Work out the finished part from the listing and answer in its coordinate system (mm). Face numbers are marked on the shaded views. A direction names the side the tool comes from. Give positions to 0.01 mm unless a question says otherwise; leave off trailing zeros. Loops run counter-clockwise (first coordinate to the right, second up) from the corner with the lowest first, then second, coordinate; pieces in that order, holes last. Notation, with made-up numbers: M 63,22 L 93,22 A24 cw 93,43 Z; hole C 13.25,31.5 d6. An arc over 180 degrees is marked long. Use a Markdown table: item, result.
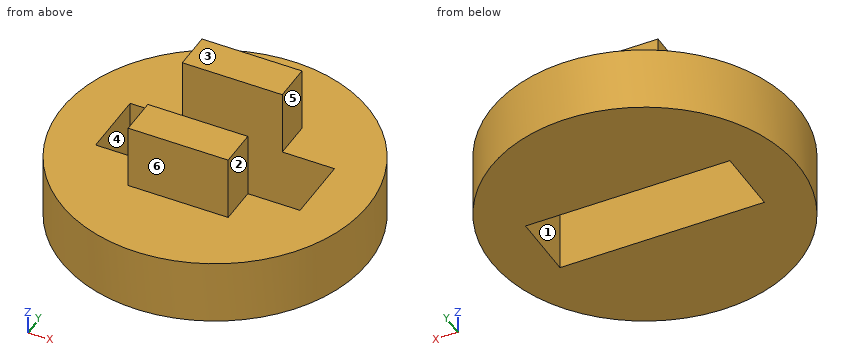
```python
from build123d import *

# Parameters (mm, degrees)
F0_R     = 59.748892
F1_DEPTH = 25.4
F2_W     = 39.043996
F2_H     = 56.034788
F3_DEPTH = 25.4
F4_W     = 21.79923
F4_H     = 26.16598
F5_DEPTH = 50.8
F6_W     = 79.802156
F6_H     = 26.16598
F7_DEPTH = 50.801


with BuildPart() as f1:
    # F0 (on Top) → F1 (new body)
    with BuildSketch(Plane.XY):
        Circle(F0_R)
    extrude(amount=F1_DEPTH)

    # F2 (on face) → F3 (join)
    with BuildSketch(Plane.XY.offset(25.4)):
        Rectangle(F2_W, F2_H)
    extrude(amount=F3_DEPTH)

    # F4 (on face) → F5 (cut, through all)
    with BuildSketch(Plane.XY.offset(50.8)):
        Rectangle(F4_W, F4_H)
    extrude(amount=-F5_DEPTH, mode=Mode.SUBTRACT)

    # F6 (on face) → F7 (cut, through all)
    with BuildSketch(Plane.XY.offset(50.8)):
        Rectangle(F6_W, F6_H)
    extrude(amount=-F7_DEPTH, mode=Mode.SUBTRACT)


solid = f1.part
```
(1) Given P1, Ø4, axis at y = -33.5, z = 23.5, coming from the +X side; P2, Ø16.5, axis at y = 17.5, z = 34, coming from the +X side; P3, Ø12, axis at y = 19, z = 41.5, coming from the -X side; P4, Ø6, axis at x = -23.5, z = 36, coming from the -Y side, each flat-ended and moving along its own axis, determine where each tip first touches the part or whether it passes through.
Entries:
| item | result |
|---|---|
| P1 | stops at x = 50.77 |
| P2 | stops at x = 19.52 |
| P3 | stops at x = -19.52 |
| P4 | passes through |
(2) A cutting plane is placed at B-B (x = 0). Write down the section's boundary in (y, z).
Entries:
| item | result |
|---|---|
| outline | M -59.75,0 L -13.08,0 L -13.08,50.8 L -28.02,50.8 L -28.02,25.4 L -59.75,25.4 Z; M 13.08,0 L 59.75,0 L 59.75,25.4 L 28.02,25.4 L 28.02,50.8 L 13.08,50.8 Z |
(3) A cutting plane is placed at A-A (y = 0). Write down the section's boundary in (x, z).
Entries:
| item | result |
|---|---|
| outline | M -59.75,0 L -39.9,0 L -39.9,25.4 L -59.75,25.4 Z; M 39.9,0 L 59.75,0 L 59.75,25.4 L 39.9,25.4 Z |
(4) The mould has two halves that part along Y. Classify the marked faces 4, 5 and 6: released by +Y, released by -Y, zero draft, split by the parting line, or undercut.
Entries:
| item | result |
|---|---|
| face 4 | undercut |
| face 5 | zero draft |
| face 6 | released by -Y |
(5) Consider probe 1 along Y at (x, z) = (3, 43); probe 2 along Z at (x, y) = (-7, 55.5); probe 3 along Y at (x, z) = (-32, 18). Determine where each line is inside the solid, lowest interval first. Write a range as [from, to].
Entries:
| item | result |
|---|---|
| probe 1 | y = [-28.02, -13.08], [13.08, 28.02] |
| probe 2 | z = [0, 25.4] |
| probe 3 | y = [-50.46, -13.08], [13.08, 50.46] |
(6) A cutting plane is placed at C-C (z = 36.5). Write down the section's boundary in (x, y).
Entries:
| item | result |
|---|---|
| outline | M -19.52,-28.02 L 19.52,-28.02 L 19.52,-13.08 L -19.52,-13.08 Z; M -19.52,13.08 L 19.52,13.08 L 19.52,28.02 L -19.52,28.02 Z |
(7) A cutting plane is placed at D-D (z = 22.5). Write down the section's boundary in (x, y), and give its area (3 significant figures).
Entries:
| item | result |
|---|---|
| outline | C 0,0 d119.5; hole M -39.9,-13.08 L 39.9,-13.08 L 39.9,13.08 L -39.9,13.08 Z |
| area | 9,130 mm² |
(8) Which of the six approach directions +Z, -Z, +X, -X, +Y, -Y give full straight-line access (tool end or side, diameter ignored) to the marked faces 1, 2 and 3?
Entries:
| item | result |
|---|---|
| face 1 | +Z, -Z |
| face 2 | +Z, +X, +Y, -Y |
| face 3 | +Z, +X, -X, +Y, -Y |
